Autodesk Inventor part; units mm, degrees
ref_plane "YZ Plane" through (0, 0, 0) normal (1, 0, 0) x (0, 1, 0)
ref_plane "XZ Plane" through (0, 0, 0) normal (0, 1, 0) x (-1, 0, 0)
ref_plane "XY Plane" through (0, 0, 0) normal (0, 0, 1) x (1, 0, 0)
sketch "Sketch1" plane through (0, 0, 0) normal (0, 0, 1) x (1, 0, 0)
  line L0 (-4, 4) -> (4, 4)
  line L1 (4, 4) -> (4, -4)
  line L2 (4, -4) -> (-4, -4)
  line L3 (-4, -4) -> (-4, 4)
  point P0 (0, 0)
  dimension "d0" = 8
  dimension "d1" = 8
  dimension "d2" = 4
  dimension "d3" = 4
extrude "Extrusion1" add sketch "Sketch1" along normal blind 3.2
shell "Shell1" thickness 1.5 removed faces 1 at (-1.3333, 1.3333, 0)
sketch "Sketch2" plane through (0, 0, 3.2) normal (0, 0, 1) x (1, 0, 0)
  circle A0 centre (0, 0) radius 2.5
  line L0 (4, 4) -> (4, -4)
  line L1 (4, -4) -> (-4, -4)
  dimension "d7" = 5
  dimension "d10" = 4
  dimension "d11" = 4
extrude "Extrusion2" add sketch "Sketch2" along normal blind 1.6
sketch "Sketch3" plane through (2.5, -2.5, 1.7) normal (0, 0, -1) x (-1, 0, 0)
  circle A0 centre (2.5, 2.5) radius 2.5
  circle A1 centre (2.5, 2.5) radius 1.2
  point P0 (2.5, 2.5)
  dimension "d18" = 2.4
extrude "Extrusion3" cut sketch "Sketch3" against normal blind 1.6 contours A1
pattern_of_one "Rectangular Pattern1"
sketch "Sketch4" plane through (2.5, -2.5, 1.7) normal (0, 0, -1) x (-1, 0, 0)
  circle A0 centre (2.5, 2.5) radius 1.2
  line L0 (0, 5) -> (0, 0)
  line L1 (0, 0) -> (5, 0)
  circle A1 centre (6.5, 6.5) radius 3.15
  circle A2 centre (6.5, 6.5) radius 2.5
  point P0 (2.5, 2.5)
  dimension "d21" = 6.5
  dimension "d22" = 6.5
  dimension "d24" = 2.5
  dimension "d25" = 5
  dimension "d26" = 6.3
extrude "Extrusion4" [suppressed]
pattern_linear "Rectangular Pattern2" [suppressed]
equation "\"d0\" = 0.8 * WIDTH"
equation "\"d1\" = 0.8 * LENGTH"
equation "\"d4\" = HEIGHT"
equation "\"d21\" = 0.5 * d23 + 0.5 * d24"
equation "\"d22\" = d21"
equation "\"WIDTH\" = 1"
equation "\"HEIGHT\" = 3.2"
properties part number "3024" material "Steel"
CAD build for the part. Positions are in the model's coordinates, mm. A direction names the side the tool comes from. Coordinates: 2 decimals unless noted, no trailing zeros. Write each loop counter-clockwise with the first axis right and the second up, starting at its lowest first coordinate (ties: lowest second). Pieces come first, ordered by that corner, then holes. Notation, with made-up numbers: M -9.5,-14.75 L 17.5,-14.75 A8 cw 17.5,-8.75 Z; hole C 61,36.5 d7. An arc over 180 degrees is marked long. Answer as a JSON object with one key per item and string values. Group by question number.
1) Pin check, flat tips, straight feed: pin 1 Ø3 at (x, y) = (1.5, -2) entering from -Z; pin 2 Ø1.4 at (x, y) = (0, 0) entering from -Z. Stop position of each tip, or through.
2) Wall check: line 1 (Y direction, x = 0, z = 2.5); line 2 (Z direction, x = 0.5, y = -1.75); line 3 (X direction, y = -1, z = 2.4). Give the ranges that are in metal, low to high. Write a range as from..to.
3) Saw through at C-C (x = 1.5). Write the cut outline in (y, z), plus the area to 3 significant figures.
4) Saw through at A-A (z = 1.5). Write the cut outline in (x, y), plus the area to 3 significant figures.
5) Saw through at B-B (y = 0). Write the cut outline in (x, z).
6) Tool access for faces 1 (the face through (0, -4, 2)), 2 (the face through (-2.5, 0, 1)): list every direction of +Z, -Z, +X, -X, +Y, -Y with a clear straight run to the whole face (end or side of a thin tool).
7) Mould opens along X. For faces 3 (the face through (-2, 2, 3.2)), 4 (the face through (-0.54, 2.44, 3.99)), 5 (the face through (0, -2.5, 1)) say: +X half, -X half, draft (parallel to the pull), parting line (faces both ways), or undercut.
Values follow:
{
 "1": {"pin 1": "stops at z = 0", "pin 2": "stops at z = 3.3"},
 "2": {"line 1": "y = -4..-1.2, 1.2..4", "line 2": "z = 1.7..4.8", "line 3": "x = -4..-0.66, 0.66..4"},
 "3": {"outline": "M -4,0 L -2.5,0 L -2.5,1.7 L 2.5,1.7 L 2.5,0 L 4,0 L 4,3.2 L 2,3.2 L 2,4.8 L -2,4.8 L -2,3.2 L -4,3.2 Z", "area": "23.5 mm2"},
 "4": {"outline": "M -4,-4 L 4,-4 L 4,4 L -4,4 Z; hole M -2.5,-2.5 L 2.5,-2.5 L 2.5,2.5 L -2.5,2.5 Z", "area": "39.0 mm2"},
 "5": {"outline": "M -4,0 L -2.5,0 L -2.5,1.7 L -1.2,1.7 L -1.2,3.3 L 1.2,3.3 L 1.2,1.7 L 2.5,1.7 L 2.5,0 L 4,0 L 4,3.2 L 2.5,3.2 L 2.5,4.8 L -2.5,4.8 L -2.5,3.2 L -4,3.2 Z"},
 "6": {"face 1": "+Z, -Z, +X, -X, -Y", "face 2": "-Z"},
 "7": {"face 3": "draft", "face 4": "parting line", "face 5": "undercut"}
}
